Solid Edge part; units mm, degrees
sketch "Sketch1" plane through (0, 0, 0) normal (0, 0, 1) x (1, 0, 0)
  circle A0 centre (6, 6) radius 2.2
  circle A1 centre (-6, -6) radius 2.2
  circle A2 centre (6, -6) radius 2.2
  line L0 (-12, 12) -> (12, 12)
  line L1 (12, 12) -> (12, -12)
  line L2 (12, -12) -> (-12, -12)
  line L3 (-12, -12) -> (-12, 12)
  circle A3 centre (-6, 6) radius 2.2
  dimension "D1" = 12
  dimension "D2" = 12
extrude "Protrusion1" add sketch "Sketch1" along normal blind 16
sketch "Sketch2" plane through (0, -12, 8) normal (0, -1, 0) x (1, 0, 0)
  line L0 (-4.2, 4.2) -> (-4.2, 14.9172)
  line L1 (4.2, 4.2) -> (4.2, 14.9172)
  arc A0 (4.2, 4.2) -> (-4.2, 4.2) centre (0, 4.2) cw
extrude "Cutout1" cut sketch "Sketch2" against normal through all material side at (-4.15, -12, 17.5586)
sketch "Sketch3" plane through (-12, -6.7, 8) normal (-1, 0, 0) x (0, -1, 0)
  line L0 (4, 7.7) -> (-4, 7.7)
extrude "Cutout2" cut sketch "Sketch3" against normal through all material side at (-12, -6.7, 15.75)
sketch "Sketch4" plane through (-12, -6.7, 7.85) normal (-1, 0, 0) x (0, -1, 0)
  line L0 (53.3, -5.85) -> (-66.7, -5.85)
extrude "Cutout3" cut sketch "Sketch4" against normal through all material side at (-12, 0, 1.95)
sketch "Sketch5" plane through (-8.1, 0, 15.7) normal (0, 0, 1) x (1, 0, 0)
  line L0 (2.1, 3.8) -> (14.1, 3.8)
  line L1 (14.1, 3.8) -> (14.1, 8.2)
  line L2 (14.1, 8.2) -> (2.1, 8.2)
  line L3 (2.1, 8.2) -> (2.1, 3.8)
  line L4 (2.1, -3.8) -> (14.1, -3.8)
  line L5 (14.1, -3.8) -> (14.1, -8.2)
  line L6 (14.1, -8.2) -> (2.1, -8.2)
  line L7 (2.1, -8.2) -> (2.1, -3.8)
extrude "Cutout4" cut sketch "Sketch5" against normal up to vertex (7.7 mm away)
properties material "ABS Plastic, medium impact"
Here's how the part is built. I have some questions about the finished solid (model axes, mm). A direction names the side the tool comes from. Round coordinates to 2 decimals unless told otherwise and drop trailing zeros. Order: outer loops, then holes, each group sorted by start corner. A loop starts at its lowest first (then second) coordinate and runs counter-clockwise, first axis right, second up. Notation, with made-up numbers: M -14.5,42 L 36.5,42 A28 cw 36.5,66 Z; hole C 53,34.5 d8. An arc over 180 degrees is marked long. Answer as CSV lines item,"result".
Item 1: Which directions (+Z, -Z, +X, -X, +Y, -Y) give clear straight access to the entire face, cutting with the end or side of a thin tool? Please do faces 1 (the flat face through (0, 6, 8)), 2 (the cylindrical face through (8.032, -5.157, 7.232)), 3 (the flat face through (-4.2, -10, 14)).
From the geometry:
face 1,"+Z"
face 2,"+Z, -Z"
face 3,"+Z, +Y, -Y"
Item 2: Imagine slicing it at D-D on x = -7.25. List the corners of the cut face in (y, z) for me, and give its area (3 significant figures).
From the geometry:
outline,"M -12,2 L -7.81,2 L -7.81,15.7 L -12,15.7 Z; M -4.19,2 L 4.19,2 L 4.19,15.7 L -4.19,15.7 Z; M 7.81,2 L 12,2 L 12,15.7 L 7.81,15.7 Z"
area,"230 mm2"
Item 3: Please list where these lines run through material, in increasing order: L1, parallel to Y at x = -6, z = 12.75; L2, parallel to X at y = 6, z = 10.5; L3, parallel to X at y = 6.5, z = 5.25. Write a range as [from, to].
From the geometry:
L1,"[-12, -8.2], [-3.8, 3.8], [8.2, 12]"
L2,"[-12, -8.2], [8.2, 12]"
L3,"[-12, -8.14], [-3.86, 3.86], [8.14, 12]"
Item 4: Imagine slicing it at C-C on z = 6.5. List the corners of the cut face in (x, y) for me, and give its area (3 significant figures).
From the geometry:
outline,"M -12,-12 L 12,-12 L 12,12 L -12,12 Z; hole C -6,-6 d4.4; hole C -6,6 d4.4; hole C 6,-6 d4.4; hole C 6,6 d4.4"
area,"515 mm2"
Item 5: For pin 1 (1.3 mm diameter, centred on x = -2, y = -6, fed in from +Z); pin 2 (3 mm diameter, centred on x = -1.5, y = -8, fed in from +Z); pin 3 (1.8 mm diameter, centred on x = -2, z = 13.5, fed in from +Y), each with a flat end and sliding along its axis, tell me the tip position at first contact or that it passes through.
From the geometry:
pin 1,"z = 8"
pin 2,"z = 9.25"
pin 3,"through"
Item 6: Imagine slicing it at B-B on y = -4.75. List the corners of the cut face in (x, z) for me.
From the geometry:
outline,"M -12,2 L -7.81,2 L -7.81,15.7 L -12,15.7 Z; M -4.19,2 L 4.19,2 L 4.19,8 L -4.19,8 Z; M 7.81,2 L 12,2 L 12,15.7 L 7.81,15.7 Z"
Item 7: Imagine slicing it at A-A on z = 13. List the corners of the cut face in (x, y) for me.
From the geometry:
outline,"M -12,-12 L -4.2,-12 L -4.2,-8.2 L -6,-8.2 A2.2 cw -6,-3.8 L -4.2,-3.8 L -4.2,3.8 L -6,3.8 A2.2 cw -6,8.2 L -4.2,8.2 L -4.2,12 L -12,12 Z; M 4.2,-12 L 12,-12 L 12,12 L 4.2,12 L 4.2,8.2 L 6,8.2 A2.2 cw 6,3.8 L 4.2,3.8 L 4.2,-3.8 L 6,-3.8 A2.2 cw 6,-8.2 L 4.2,-8.2 Z"
Item 8: We'd pull the mould along Y, two halves only. Please class faces 4 (the cylindrical face through (0, 0, 8)), 5 (the cylindrical face through (8.032, 6.843, 7.232)): +Y half, -Y half, draft (parallel to the pull), parting line (faces both ways), or undercut.
From the geometry:
face 4,"draft"
face 5,"undercut"
